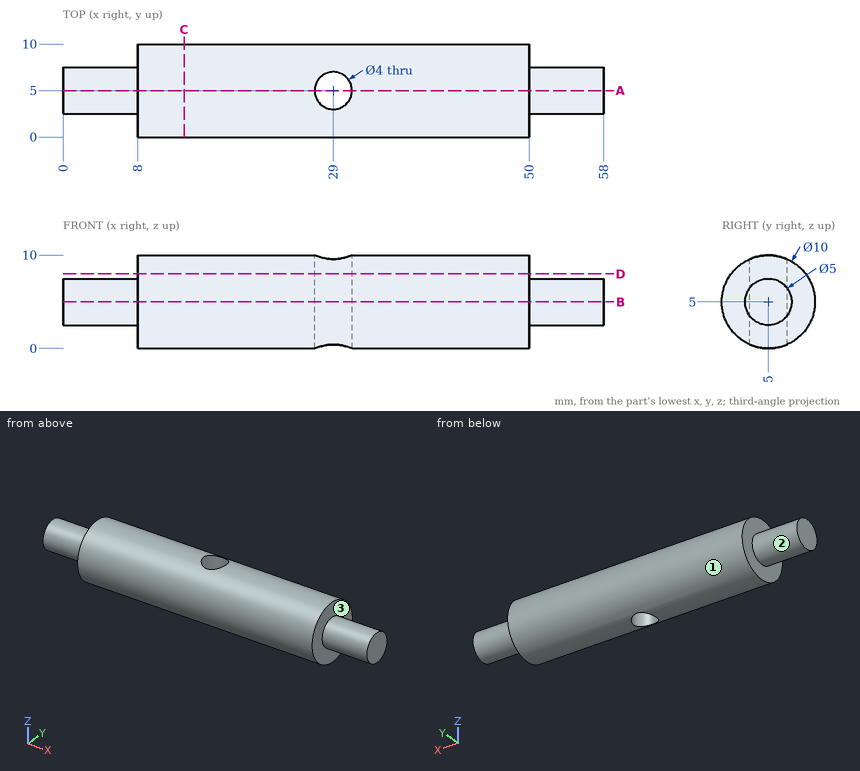
Can you work these out from the drawing? Everything is in mm from the part's minimum corner. A direction names the side the tool comes from. Coordinates: 2 decimals unless noted, no trailing zeros. Loops run counter-clockwise (first coordinate to the right, second up) from the corner with the lowest first, then second, coordinate; pieces in that order, holes last.
1. Imagine slicing it at A-A, the plane y = 5. Please give me the cut outline in (x, z).
2. Imagine slicing it at B-B, the plane z = 5. Please give me the cut outline in (x, y), and give its area (3 significant figures).
3. Imagine slicing it at C-C, the plane x = 13. Please give me the cut outline in (y, z), and give its area (3 significant figures).
4. Imagine slicing it at D-D, the plane z = 8. Please give me the cut outline in (x, y).
5. I need wall thicknesses on L1, parallel to X at y = 7.5, z = 4; L2, parallel to Y at x = 29, z = 4.25; L3, parallel to Y at x = 29, z = 3. Which ranges of each line are inside material? Lowest first, please.
6. For P1, Ø5, axis at y = 3, z = 7.5, coming from the -X side; P2, Ø4, axis at y = 8, z = 9, coming from the -X side; P3, Ø1, axis at x = 37.5, z = 4, coming from the -Y side; P4, Ø2, axis at x = 8.5, z = 2, coming from the -Y side, each with a flat end and sliding along its axis, tell me the tip position at first contact or that it passes through.
7. For the marked faces 1, 2 and 3, which set-ups out of +Z, -Z, +X, -X, +Y, -Y let a thin tool reach every point of the face, with its end or its side?
Taken from the geometry:
1. outline: (0, 2.5) - (8, 2.5) - (8, 0) - (27, 0) - (27, 10) - (8, 10) - (8, 7.5) - (0, 7.5) - close; (31, 0) - (50, 0) - (50, 2.5) - (58, 2.5) - (58, 7.5) - (50, 7.5) - (50, 10) - (31, 10) - close
2. outline: (0, 2.5) - (8, 2.5) - (8, 0) - (50, 0) - (50, 2.5) - (58, 2.5) - (58, 7.5) - (50, 7.5) - (50, 10) - (8, 10) - (8, 7.5) - (0, 7.5) - close; hole circle Ø4 at (29, 5)
2. area: 487 mm2
3. outline: circle Ø10 at (5, 5)
3. area: 78.5 mm2
4. outline: (8, 1) - (50, 1) - (50, 9) - (8, 9) - close; hole circle Ø4 at (29, 5)
5. L1: x = 8 to 50
5. L2: y = 0.06 to 3, 7 to 9.94
5. L3: y = 0.42 to 3, 7 to 9.58
6. P1: stops at x = 0
6. P2: stops at x = 8
6. P3: stops at y = 0.03
6. P4: stops at y = 0.42
7. face 1: +X, -X
7. face 2: -X
7. face 3: +X
